Autodesk Inventor part; units mm, degrees
ref_plane "BoardFrontPlane" through (0, 0, 0) normal (0, 0, 1) x (1, 0, 0)
ref_plane "YZ Plane" through (0, 0, 0) normal (1, 0, 0) x (0, 1, 0)
ref_plane "XZ Plane" through (0, 0, 0) normal (0, 1, 0) x (-1, 0, 0)
ref_plane "BoardFrontPlane" through (0, 0, 0) normal (0, 0, 1) x (1, 0, 0)
sketch "Sketch1" plane through (0, 0, 0) normal (0, 0, 1) x (1, 0, 0)
  line L0 (149.925, 120.925) -> (241.925, 120.925)
  line L1 (241.925, 120.925) -> (241.925, 160.925)
  line L2 (241.925, 160.925) -> (149.925, 160.925)
  line L3 (149.925, 160.925) -> (149.925, 120.925)
extrude "BoardOutline" add sketch "Sketch1" along normal blind 1.5954
sketch "Sketch4" plane through (0, 0, 1.5954) normal (0, 0, 1) x (1, 0, 0)
  point P0 (219.993, 140.177)
hole "U1-1" at (219.993, 140.177, 1.5954) direction (0, 0, -1) diameter 1.5 end through all
sketch "Sketch5" plane through (0, 0, 1.5954) normal (0, 0, 1) x (1, 0, 0)
  point P0 (225.073, 153.027)
hole "U1-4" at (225.073, 153.027, 1.5954) direction (0, 0, -1) diameter 1.5 end through all
sketch "Sketch6" plane through (0, 0, 1.5954) normal (0, 0, 1) x (1, 0, 0)
  point P0 (225.073, 146.527)
hole "U1-3" at (225.073, 146.527, 1.5954) direction (0, 0, -1) diameter 1.5 end through all
sketch "Sketch7" plane through (0, 0, 1.5954) normal (0, 0, 1) x (1, 0, 0)
  point P0 (197.073, 157.127)
hole "U1-5" at (197.073, 157.127, 1.5954) direction (0, 0, -1) diameter 1.5 end through all
sketch "Sketch8" plane through (0, 0, 1.5954) normal (0, 0, 1) x (1, 0, 0)
  point P0 (197.073, 149.507)
hole "U1-6" at (197.073, 149.507, 1.5954) direction (0, 0, -1) diameter 1.5 end through all
sketch "Sketch9" plane through (0, 0, 1.5954) normal (0, 0, 1) x (1, 0, 0)
  point P0 (225.073, 140.127)
hole "U1-2" at (225.073, 140.127, 1.5954) direction (0, 0, -1) diameter 1.5 end through all
sketch "Sketch10" plane through (0, 0, 1.5954) normal (0, 0, 1) x (1, 0, 0)
  point P0 (155.425, 126.225)
hole "SW1-1" at (155.425, 126.225, 1.5954) direction (0, 0, -1) diameter 0.9 end through all
sketch "Sketch11" plane through (0, 0, 1.5954) normal (0, 0, 1) x (1, 0, 0)
  point P0 (157.925, 126.225)
hole "SW1-2" at (157.925, 126.225, 1.5954) direction (0, 0, -1) diameter 0.9 end through all
sketch "Sketch12" plane through (0, 0, 1.5954) normal (0, 0, 1) x (1, 0, 0)
  point P0 (160.425, 126.225)
hole "SW1-3" at (160.425, 126.225, 1.5954) direction (0, 0, -1) diameter 0.9 end through all
sketch "Sketch13" plane through (0, 0, 1.5954) normal (0, 0, 1) x (1, 0, 0)
  point P0 (157.925, 131.625)
hole "SW1-5" at (157.925, 131.625, 1.5954) direction (0, 0, -1) diameter 0.9 end through all
sketch "Sketch14" plane through (0, 0, 1.5954) normal (0, 0, 1) x (1, 0, 0)
  point P0 (160.425, 131.625)
hole "SW1-6" at (160.425, 131.625, 1.5954) direction (0, 0, -1) diameter 0.9 end through all
sketch "Sketch15" plane through (0, 0, 1.5954) normal (0, 0, 1) x (1, 0, 0)
  point P0 (155.425, 131.625)
hole "SW1-4" at (155.425, 131.625, 1.5954) direction (0, 0, -1) diameter 0.9 end through all
sketch "Sketch16" plane through (0, 0, 1.5954) normal (0, 0, 1) x (1, 0, 0)
  point P0 (160.925, 128.925)
hole "SW1-0" at (160.925, 128.925, 1.5954) direction (0, 0, -1) diameter 1.2 end through all
sketch "Sketch22" plane through (0, 0, 1.5954) normal (0, 0, 1) x (1, 0, 0)
  point P0 (156.175, 143.45)
hole "CN2-1" at (156.175, 143.45, 1.5954) direction (0, 0, -1) diameter 0.72 end through all
sketch "Sketch23" plane through (0, 0, 1.5954) normal (0, 0, 1) x (1, 0, 0)
  point P0 (156.175, 149.45)
hole "CN2-4" at (156.175, 149.45, 1.5954) direction (0, 0, -1) diameter 0.72 end through all
sketch "Sketch24" plane through (0, 0, 1.5954) normal (0, 0, 1) x (1, 0, 0)
  point P0 (156.175, 145.45)
hole "CN2-2" at (156.175, 145.45, 1.5954) direction (0, 0, -1) diameter 0.72 end through all
sketch "Sketch25" plane through (0, 0, 1.5954) normal (0, 0, 1) x (1, 0, 0)
  point P0 (156.175, 151.45)
hole "CN2-5" at (156.175, 151.45, 1.5954) direction (0, 0, -1) diameter 0.72 end through all
sketch "Sketch26" plane through (0, 0, 1.5954) normal (0, 0, 1) x (1, 0, 0)
  point P0 (156.175, 147.45)
hole "CN2-3" at (156.175, 147.45, 1.5954) direction (0, 0, -1) diameter 0.72 end through all
sketch "Sketch27" plane through (0, 0, 1.5954) normal (0, 0, 1) x (1, 0, 0)
  point P0 (156.175, 153.45)
hole "CN2-6" at (156.175, 153.45, 1.5954) direction (0, 0, -1) diameter 0.72 end through all
sketch "Sketch28" plane through (0, 0, 1.5954) normal (0, 0, 1) x (1, 0, 0)
  point P0 (231.2, 150.95)
hole "CN1-1" at (231.2, 150.95, 1.5954) direction (0, 0, -1) diameter 1.9 end through all
sketch "Sketch29" plane through (0, 0, 1.5954) normal (0, 0, 1) x (1, 0, 0)
  point P0 (231.2, 142.69)
hole "CN1-2" at (231.2, 142.69, 1.5954) direction (0, 0, -1) diameter 1.9 end through all
sketch "Sketch30" plane through (0, 0, 1.5954) normal (0, 0, 1) x (1, 0, 0)
  point P0 (213.725, 126.35)
hole "C2-1" at (213.725, 126.35, 1.5954) direction (0, 0, -1) diameter 0.8 end through all
sketch "Sketch31" plane through (0, 0, 1.5954) normal (0, 0, 1) x (1, 0, 0)
  point P0 (213.725, 131.35)
hole "C2-2" at (213.725, 131.35, 1.5954) direction (0, 0, -1) diameter 0.8 end through all
sketch "Sketch32" plane through (0, 0, 1.5954) normal (0, 0, 1) x (1, 0, 0)
  point P0 (204.925, 128.925)
hole "CN3-1" at (204.925, 128.925, 1.5954) direction (0, 0, -1) diameter 1 end through all
sketch "Sketch33" plane through (0, 0, 1.5954) normal (0, 0, 1) x (1, 0, 0)
  point P0 (199.845, 134.005)
hole "CN3-2_KIXDPQYP" at (199.845, 134.005, 1.5954) direction (0, 0, -1) diameter 2.64 end through all
sketch "Sketch34" plane through (0, 0, 1.5954) normal (0, 0, 1) x (1, 0, 0)
  point P0 (210.005, 123.845)
hole "CN3-2_CBVBVUTG" at (210.005, 123.845, 1.5954) direction (0, 0, -1) diameter 2.64 end through all
sketch "Sketch35" plane through (0, 0, 1.5954) normal (0, 0, 1) x (1, 0, 0)
  point P0 (204.925, 126.385)
hole "CN3-2_RGICKRHG" at (204.925, 126.385, 1.5954) direction (0, 0, -1) diameter 1 end through all
sketch "Sketch36" plane through (0, 0, 1.5954) normal (0, 0, 1) x (1, 0, 0)
  point P0 (239.425, 158.425)
hole "Free-0_VQVYAAFI" at (239.425, 158.425, 1.5954) direction (0, 0, -1) diameter 3.2 end through all
sketch "Sketch37" plane through (0, 0, 1.5954) normal (0, 0, 1) x (1, 0, 0)
  point P0 (152.425, 123.425)
hole "Free-0_TSXFHYQJ" at (152.425, 123.425, 1.5954) direction (0, 0, -1) diameter 3.2 end through all
sketch "Sketch38" plane through (0, 0, 1.5954) normal (0, 0, 1) x (1, 0, 0)
  point P0 (152.425, 158.425)
hole "Free-0_JLGAYVLC" at (152.425, 158.425, 1.5954) direction (0, 0, -1) diameter 3.2 end through all
sketch "Sketch54" plane through (0, 0, 1.5954) normal (0, 0, 1) x (1, 0, 0)
  line L0 (181.425, 133.3251) -> (181.425, 134.1251) construction
  line L1 (181.925, 133.3251) -> (181.925, 134.1251)
  line L2 (180.925, 134.1251) -> (180.925, 133.3251)
  arc A0 (180.925, 133.3251) -> (181.925, 133.3251) centre (181.425, 133.3251) ccw
  arc A1 (181.925, 134.1251) -> (180.925, 134.1251) centre (181.425, 134.1251) ccw
  point P0 (181.425, 133.7251)
extrude "R3-0_UKQXETQG" cut sketch "Sketch54" against normal through all
sketch "Sketch55" plane through (0, 0, 1.5954) normal (0, 0, 1) x (1, 0, 0)
  line L0 (181.425, 123.7251) -> (181.425, 124.5251) construction
  line L1 (181.925, 123.7251) -> (181.925, 124.5251)
  line L2 (180.925, 124.5251) -> (180.925, 123.7251)
  arc A0 (180.925, 123.7251) -> (181.925, 123.7251) centre (181.425, 123.7251) ccw
  arc A1 (181.925, 124.5251) -> (180.925, 124.5251) centre (181.425, 124.5251) ccw
  point P0 (181.425, 124.1251)
extrude "R3-0_WDTRLAVX" cut sketch "Sketch55" against normal through all
sketch "Sketch56" plane through (0, 0, 1.5954) normal (0, 0, 1) x (1, 0, 0)
  line L0 (173.925, 131.19) -> (173.925, 131.6601) construction
  line L1 (174.325, 131.19) -> (174.325, 131.6601)
  line L2 (173.525, 131.6601) -> (173.525, 131.19)
  arc A0 (173.525, 131.19) -> (174.325, 131.19) centre (173.925, 131.19) ccw
  arc A1 (174.325, 131.6601) -> (173.525, 131.6601) centre (173.925, 131.6601) ccw
  point P0 (173.925, 131.425)
extrude "R3-1" cut sketch "Sketch56" against normal through all
sketch "Sketch57" plane through (0, 0, 1.5954) normal (0, 0, 1) x (1, 0, 0)
  line L0 (173.925, 126.1901) -> (173.925, 126.6601) construction
  line L1 (174.325, 126.1901) -> (174.325, 126.6601)
  line L2 (173.525, 126.6601) -> (173.525, 126.1901)
  arc A0 (173.525, 126.1901) -> (174.325, 126.1901) centre (173.925, 126.1901) ccw
  arc A1 (174.325, 126.6601) -> (173.525, 126.6601) centre (173.925, 126.6601) ccw
  point P0 (173.925, 126.4251)
extrude "R3-3" cut sketch "Sketch57" against normal through all
sketch "Sketch58" plane through (0, 0, 1.5954) normal (0, 0, 1) x (1, 0, 0)
  line L0 (173.925, 128.69) -> (173.925, 129.1601) construction
  line L1 (174.325, 128.69) -> (174.325, 129.1601)
  line L2 (173.525, 129.1601) -> (173.525, 128.69)
  arc A0 (173.525, 128.69) -> (174.325, 128.69) centre (173.925, 128.69) ccw
  arc A1 (174.325, 129.1601) -> (173.525, 129.1601) centre (173.925, 129.1601) ccw
  point P0 (173.925, 128.925)
extrude "R3-2" cut sketch "Sketch58" against normal through all
sketch "img_Top" plane through (0, 0, 1.5954) normal (0, 0, 1) x (1, 0, 0)
  line L0 (149.925, 160.925) -> (241.925, 160.925) construction
  line L1 (241.925, 160.925) -> (241.925, 120.9195) construction
  line L2 (241.925, 120.9195) -> (149.925, 120.9195) construction
  line L3 (149.925, 120.9195) -> (149.925, 160.925) construction
decal "Decal_Top"
sketch "img_Bottom" plane through (0, 0, -1.5954) normal (0, 0, -1) x (1, 0, 0)
  line L0 (149.925, -120.925) -> (241.925, -120.925) construction
  line L1 (241.925, -120.925) -> (241.925, -160.9305) construction
  line L2 (241.925, -160.9305) -> (149.925, -160.9305) construction
  line L3 (149.925, -160.9305) -> (149.925, -120.925) construction
decal "Decal_Bottom"
properties part number "Monitor_Blanking_V3_BOARD"
Verification items for the finished model (mm, model axes). Round coordinates to 2 decimals unless told otherwise and drop trailing zeros. Write each question's results on one line, items separated by ' | '. Start each with the question number.
1. Cross-section at A-A (z = 1.15). Count the separate pieces of the cut face and the enclosed holes in it, then the cut area to 3 significant figures.
2. Draft check along X on faces 1 (the flat face through (149.925, 141, 1)), 2 (the flat face through (195, 141, 1.595)), 3 (the cylindrical face through (208.89, 123.14, 0.79)), 4 (the cylindrical face through (238.08, 157.56, 0.79)). Enter one of: +X half, -X half, draft (parallel to the pull), parting line (faces both ways), or undercut.
3. Depth check by flat-ended pin: P1, Ø1.2, axis at x = 225.073, y = 140.127, coming from the +Z side. Enter the tip coordinate at first touch or a pass-through.
4. Material ranges on probe 1 along X at (y, z) = (142.5, 0.4) (3 decimals); probe 2 along X at (y, z) = (149.5, 0.75) (3 decimals); probe 3 along X at (y, z) = (132, 1) (3 decimals), recorded low to high. Write a range as from..to.
Solutions:
1) separate pieces: 1 | enclosed holes: 35 | area: 3,610 mm2
2) face 1: -X half | face 2: draft | face 3: undercut | face 4: undercut
3) P1: passes through
4) probe 1: x = 149.925..230.269, 232.131..241.925 | probe 2: x = 149.925..155.818, 156.532..196.323, 197.823..241.925 | probe 3: x = 149.925..155.176, 155.674..157.676, 158.174..160.176, 160.674..173.714, 174.136..241.925
